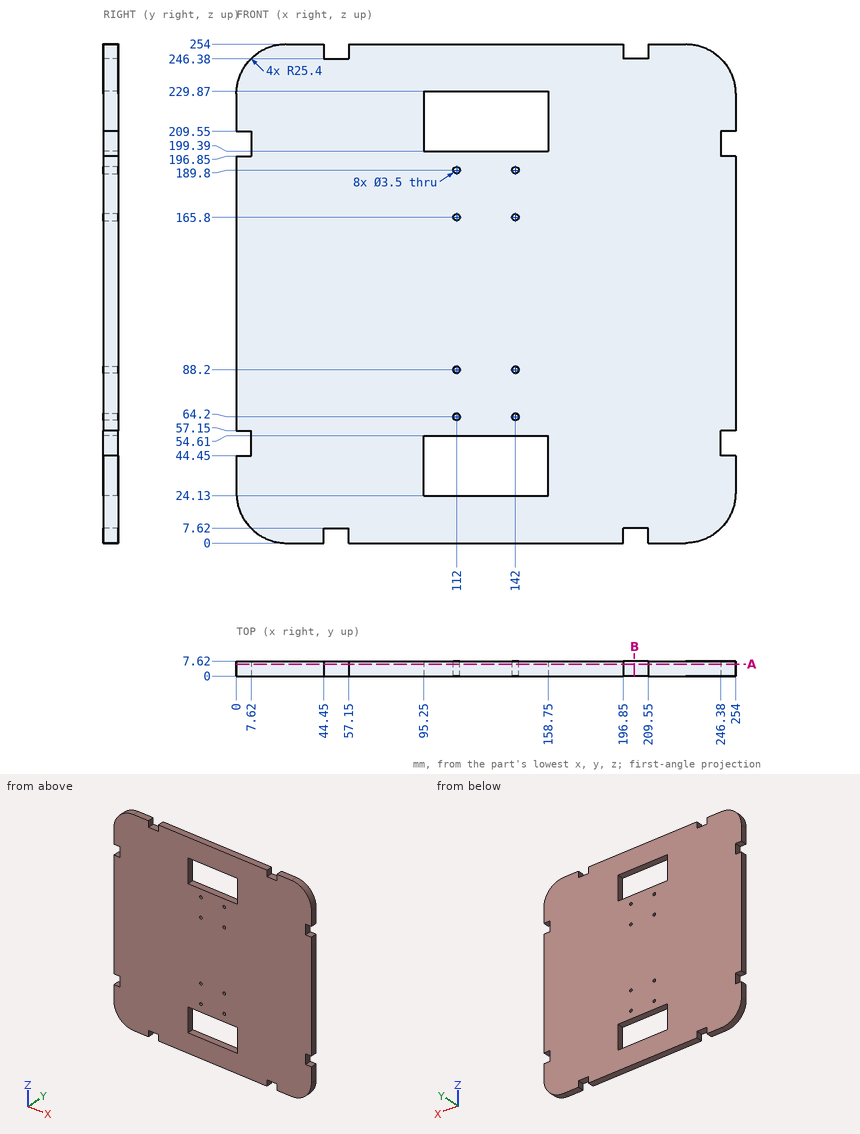
Input: dimensioned drawing with shaded views. Units: mm. Origin: part minimum x, y, z. Round coordinates to 2 decimals unless told otherwise and drop trailing zeros. Order: outer loops, then holes, each group sorted by start corner. A loop starts at its lowest first (then second) coordinate and runs counter-clockwise, first axis right, second up. Notation, with made-up numbers: (52.5, -15.75) -> (60.5, -15.75) arc R6 cw to (60.5, -11.75) -> close; hole circle Ø10 at (-29.75, -19.75). An arc over 180 degrees is marked (long way). One line per item, written item: value. Start each with the question number.
Q1. Material intervals for probe 1 along X at (y, z) = (2.5, 88.2); probe 2 along Z at (x, y) = (103.5, 7); probe 3 along X at (y, z) = (4.5, 226.5), sorted ascending.
Q2. Section query A-A (y = 6). Give the number of separate pieces and of enclosed holes in the cut face, plus the area to 3 significant figures.
Q3. Section query B-B (x = 202.5). Return the cut outline in (y, z).
Q4. Pin query (flat end, axial travel): pin 1 (3 mm diameter, centred on x = 142, z = 64.2, fed in from -Y); pin 2 (2.5 mm diameter, centred on y = 5.5, z = 3, fed in from +X); pin 3 (2.5 mm diameter, centred on x = 5, y = 3.5, fed in from -Z); pin 4 (4 mm diameter, centred on x = 50, y = 2, fed in from -Z). Return the tip coordinate at first contact, or that it passes through.
Findings below:
1. probe 1: 0 to 110.25, 113.75 to 140.25, 143.75 to 254
1. probe 2: 0 to 24.13, 54.61 to 199.39, 229.87 to 254
1. probe 3: 0 to 95.25, 158.75 to 254
2. separate pieces: 1
2. enclosed holes: 10
2. area: 59,200 mm²
3. outline: (0, 7.62) -> (7.62, 7.62) -> (7.62, 246.38) -> (0, 246.38) -> close
4. pin 1: through
4. pin 2: x = 242.67
4. pin 3: z = 8.71
4. pin 4: z = 7.62
